CAD build for the part. Positions are in the model's coordinates, mm. Coordinates: 2 decimals unless noted, no trailing zeros. Order: outer loops, then holes, each group sorted by start corner. A loop starts at its lowest first (then second) coordinate and runs counter-clockwise, first axis right, second up. Notation, with made-up numbers: M 80,-12 L 85,-12 A20 ccw 85,14 Z; hole C 36,48.5 d7. An arc over 180 degrees is marked long. Write item = value, one per line.
from build123d import *

# Parameters (mm, degrees)
SKETCH1_W                    = 31.75
SKETCH1_H                    = 31.75
BOSS_EXTRUDE1_DEPTH          = 3.175
X_0_397_DIAMETER_HOLE1_D     = 10.0838
X_0_397_DIAMETER_HOLE1_DEPTH = 12.7
X_0_397_DIAMETER_HOLE1_TIP   = 3.029479155
CIRPATTERN1_COUNT            = 4
CIRPATTERN2_COUNT            = 4


with BuildPart() as part:
    # Sketch1 → Boss-Extrude1 (new body)
    with BuildSketch(Plane(origin=(0, 0, 0), x_dir=(0, 0, -1), z_dir=(1, 0, 0))):
        Rectangle(SKETCH1_W, SKETCH1_H)
    extrude(amount=BOSS_EXTRUDE1_DEPTH)

    # X (0.397) Diameter Hole1
    with Locations(Plane(origin=(3.175, 0, 0), x_dir=(0, 0, -1), z_dir=(1, 0, 0))):
        with Locations((0, 0)):
            Hole(X_0_397_DIAMETER_HOLE1_D / 2, depth=X_0_397_DIAMETER_HOLE1_DEPTH)
            with Locations((0, 0, -(X_0_397_DIAMETER_HOLE1_DEPTH + X_0_397_DIAMETER_HOLE1_TIP / 2))):  # 118° drill point
                Cone(0, X_0_397_DIAMETER_HOLE1_D / 2, X_0_397_DIAMETER_HOLE1_TIP, mode=Mode.SUBTRACT)

    # Sketch4 → #2-56 Tapped Hole1 (revolve, cut)
    with BuildSketch(Plane(origin=(3.175, 7.4, 0), x_dir=(0, 0, -1), z_dir=(0, 1, 0))):
        Polygon((0, 0), (0, 7.13816509), (0.889, 6.604), (0.889, 0), align=None)
    f_2_56_tapped_hole1 = revolve(axis=Axis((9.525, 7.4, 0), (-1, 0, 0)), mode=Mode.SUBTRACT)

    # CirPattern1: #2-56 Tapped Hole1 ×4 about axis
    cirpattern1_axis = Axis((0, 0, 0), (1, 0, 0))
    for i in range(1, CIRPATTERN1_COUNT):
        add(f_2_56_tapped_hole1.rotate(cirpattern1_axis, i * 360 / CIRPATTERN1_COUNT), mode=Mode.SUBTRACT)

    # Sketch6 → #4-40 Tapped Hole1 (revolve, cut)
    with BuildSketch(Plane(origin=(3.175, 13.470384182, 13.470384182), x_dir=(0, 0, -1), z_dir=(0, 1, 0))):
        Polygon((0, 0), (0, 9.569152758), (1.1303, 8.89), (1.1303, 0), align=None)
    f_4_40_tapped_hole1 = revolve(axis=Axis((9.525, 13.470384182, 13.470384182), (-1, 0, 0)), mode=Mode.SUBTRACT)

    # CirPattern2: #4-40 Tapped Hole1 ×4 about axis
    cirpattern2_axis = Axis((0, 0, 0), (1, 0, 0))
    for i in range(1, CIRPATTERN2_COUNT):
        add(f_4_40_tapped_hole1.rotate(cirpattern2_axis, i * 360 / CIRPATTERN2_COUNT), mode=Mode.SUBTRACT)


solid = part.part
(1) Slice it at A-A, the plane y = 7.4. Write the cut outline in (x, z) (3 decimals).
Evaluation:
outline = M 0,-15.875 L 3.175,-15.875 L 3.175,-0.889 L 0,-0.889 Z; M 0,0.889 L 3.175,0.889 L 3.175,15.875 L 0,15.875 Z
(2) Slice it at B-B, the plane z = 0. Write the cut outline in (x, y) (3 decimals).
Evaluation:
outline = M 0,-15.875 L 3.175,-15.875 L 3.175,-8.289 L 0,-8.289 Z; M 0,-6.511 L 3.175,-6.511 L 3.175,-5.042 L 0,-5.042 Z; M 0,5.042 L 3.175,5.042 L 3.175,6.511 L 0,6.511 Z; M 0,8.289 L 3.175,8.289 L 3.175,15.875 L 0,15.875 Z
(3) Pull direction Y, two halves, no side cores. Call faces 1 (the face through (0, 4, 4)), 2 (the face through (1.61, 8.19, -0.41)), 3 (the face through (2, -15.875, 0)): +Y half, -Y half, draft (parallel to the pull), parting line (faces both ways), or undercut.
Evaluation:
face_1 = draft
face_2 = undercut
face_3 = -Y half
(4) Slice it at D-D, the plane x = 2. State how many separate pieces and enclosed holes the cut face has, then the cut area to 3 significant figures.
Evaluation:
separate_pieces = 1
enclosed_holes = 9
area = 902 mm²
(5) Wall check: line 1 (Y direction, x = 1.45, z = 0) (3 decimals); line 2 (Y direction, x = 0.5, z = -7.5) (3 decimals). Give the ranges that are in metal, low to high. Write a range as from..to.
Evaluation:
line_1 = -15.875..-8.289, -6.511..-5.042, 5.042..6.511, 8.289..15.875
line_2 = -15.875..-0.883, 0.883..15.875
